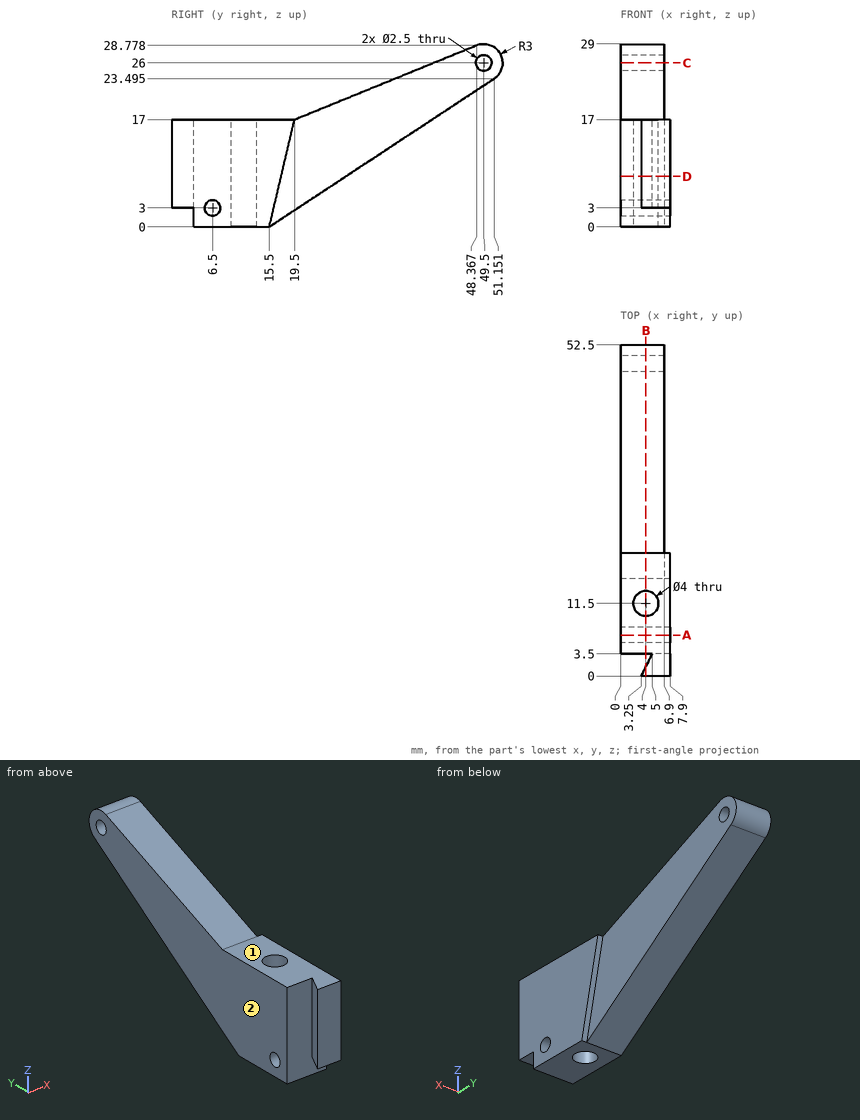
Print and shaded views of the part. All mm, measured from the part's lowest x, y and z. A direction names the side the tool comes from. Round coordinates to 2 decimals unless told otherwise and drop trailing zeros. Write each loop counter-clockwise with the first axis right and the second up, starting at its lowest first coordinate (ties: lowest second). Pieces come first, ordered by that corner, then holes.
(1) Probe line 1 along Y through (x, z) = (4, 5.5) (1 decimal); line 2 along Z through (x, y) = (0.75, 5); line 3 along Y through (x, z) = (3.5, 10.75) (1 decimal). List the from-to ranges inside material, lowest first.
(2) Drop flat-ended pins along their axis: P1, Ø4, axis at x = 4.5, y = 12.5, coming from the +Z side; P2, Ø1, axis at x = 3, y = 36, coming from the +Z side; P3, Ø1, axis at x = 1, z = 8.5, coming from the +Y side (1 decimal); P4, Ø3, axis at x = 1.5, y = 8.5, coming from the -Z side. Give the stop position or say it passes through.
(3) 3-axis set-ups, long thin cutter, end or side, ignore diameter. For the marked faces 1 and 2: which of +Z, -Z, +X, -X, +Y, -Y reach the whole face in a straight line?
(4) Slice it at C-C, the plane z = 26. Write the cut outline in (x, y).
(5) Slice it at A-A, the plane y = 6.5. Write the cut outline in (x, z).
(6) Slice it at D-D, the plane z = 8. Write the cut outline in (x, y).
(7) Slice it at B-B, the plane x = 4. Count the separate pieces of the cut face and the enclosed holes in it, and give its area (3 significant figures).
From the geometry:
1. line 1: y = 0 to 1.5, 3.5 to 9.5, 13.5 to 23.8
1. line 2: z = 0 to 17
1. line 3: y = 0 to 0.5, 3.5 to 9.6, 13.4 to 31.8
2. P1: stops at z = 17
2. P2: stops at z = 23.94
2. P3: stops at y = 29.2
2. P4: stops at z = 0
3. face 1: +Z, +X, -X, -Y
3. face 2: +Z, -Z, -X, +Y, -Y
4. outline: (0, 41.56) - (6.9, 41.56) - (6.9, 48.25) - (0, 48.25) - close; (0, 50.75) - (6.9, 50.75) - (6.9, 52.5) - (0, 52.5) - close
5. outline: (0, 0) - (7.9, 0) - (7.9, 1.75) - (0, 1.75) - close; (0, 4.25) - (7.9, 4.25) - (7.9, 17) - (0, 17) - close
6. outline: (0, 3.5) - (5, 3.5) - (3.25, 0) - (7.9, 0) - (7.9, 17.38) - (6.9, 17.38) - (6.9, 27.64) - (0, 27.64) - close; hole circle Ø4 at (4, 11.5)
7. separate pieces: 3
7. enclosed holes: 2
7. area: 542 mm2
